```python
from build123d import *

# Parameters (mm, degrees)
F2_R     = 7.2342106025
F3_DEPTH = 25
F4_R     = 3
F5_SIZE  = 2


with BuildPart() as f1:
    # F0 (on Front) → F1 (revolve)
    with BuildSketch(Plane.XZ):
        Polygon((0, 25.867851451), (0, 17.7663322538), (13.6637529358, 17.7663322538), (13.6637529358, 25.867851451), (9.3429423869, 25.867851451), (9.3429423869, 50.1724109054), (22.035324946, 50.1724109054), (22.035324946, 63.9449954033), (0, 63.9449954033), (0, 50.1724109054), (3.4018275328, 50.1724109054), (3.4018275328, 25.867851451), align=None)
    revolve(axis=Axis((6.8318764679, 0, 0), (1, 0, 0)))

    # F2 (on face) → F3 (cut)
    with BuildSketch(Plane.YZ.offset(9.3429423869)):
        with Locations((0, 36.9940809906)):
            Circle(F2_R)
        with Locations((-21.7445752284, -29.9288402126)):
            Circle(F2_R)
        with Locations((21.7445752284, -29.9288402126)):
            Circle(F2_R)
        with Locations((35.1834617904, 11.4317997174)):
            Circle(F2_R)
        with Locations((-35.1834617904, 11.4317997174)):
            Circle(F2_R)
    extrude(amount=-F3_DEPTH, mode=Mode.SUBTRACT)

    # F4
    f4_edges = [f1.edges().sort_by_distance(p)[0] for p in [
        (22.035325, 0, -63.944995),
        (0, 0, -63.944995),
        (0, 0, -50.172411),
    ]]
    fillet(f4_edges, radius=F4_R)

    # F5
    f5_edges = [f1.edges().sort_by_distance(p)[0] for p in [
        (3.401828, -7.234211, 36.994081),
        (9.342942, 27.949251, 11.4318),
        (6.372385, 42.417672, 11.4318),
        (3.401828, 27.949251, 11.4318),
        (9.342942, -42.417672, 11.4318),
        (6.372385, -27.949251, 11.4318),
        (3.401828, -42.417672, 11.4318),
        (9.342942, -28.978786, -29.92884),
        (6.372385, -14.510365, -29.92884),
        (3.401828, -28.978786, -29.92884),
        (3.401828, 14.510365, -29.92884),
    ]]
    chamfer(f5_edges, length=F5_SIZE)


solid = f1.part
```
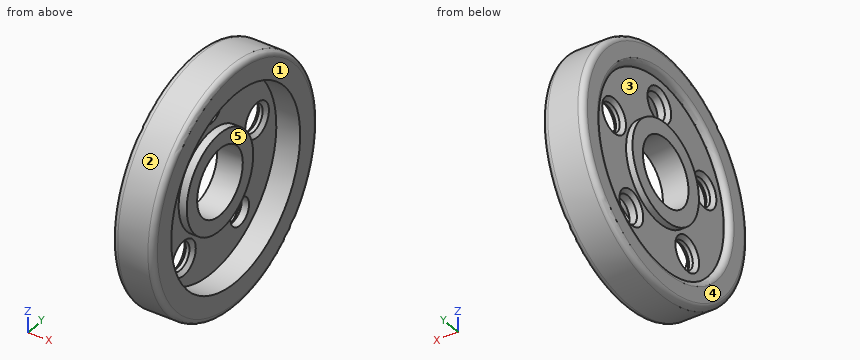
Build history of the part. All positions in model axes, mm. Face numbers are marked on the shaded views. A direction names the side the tool comes from. Give positions to 0.01 mm unless a question says otherwise; leave off trailing zeros.
1) Probe line 1 along Z through (x, y) = (7.55, 0) (3 decimals); line 2 along Z through (x, y) = (3.15, 0) (3 decimals); line 3 along Z through (x, y) = (14.25, 0) (3 decimals). List the from-to ranges inside material, lowest first.
Values follow:
line 1: z = -63.945 to -17.766, 17.766 to 29.76, 44.228 to 63.945
line 2: z = -63.945 to -50.172, -25.868 to -17.766, 17.766 to 25.868, 50.172 to 63.945
line 3: z = -63.945 to -50.172, 50.172 to 63.945
2) 3-axis set-ups, long thin cutter, end or side, ignore diameter. For the marked faces 4 and 5: which of +Z, -Z, +X, -X, +Y, -Y reach the whole face in a straight line?
Values follow:
face 4: +Z, -Z, -X, +Y, -Y
face 5: +X
3) Drop flat-ended pins along their axis: P1, Ø2, axis at x = 16.5, z = -30, coming from the -Y side; P2, Ø10, axis at x = 19, y = 34, coming from the -Z side; P3, Ø12, axis at x = 16, z = 49.5, coming from the -Y side; P4, Ø11.5, axis at y = 21.74, z = -29.93, coming from the +X side. Give the stop position or say it passes through.
Values follow:
P1: stops at y = -56.99
P2: stops at z = -56.99
P3: stops at y = -46.87
P4: passes through
4) Two-plate mould, pull along Z, no slides. Class the marked faces 1, 2 and 3: released by +Z, released by -Z, zero draft, split by the parting line, or undercut.
Values follow:
face 1: zero draft
face 2: split by the parting line
face 3: undercut
5) Band-saw the part on B-B on y = 0. State how many separate pieces and enclosed holes the cut face has, then the cut area to 3 significant figures.
Values follow:
separate pieces: 3
enclosed holes: 0
area: 1,020 mm2
